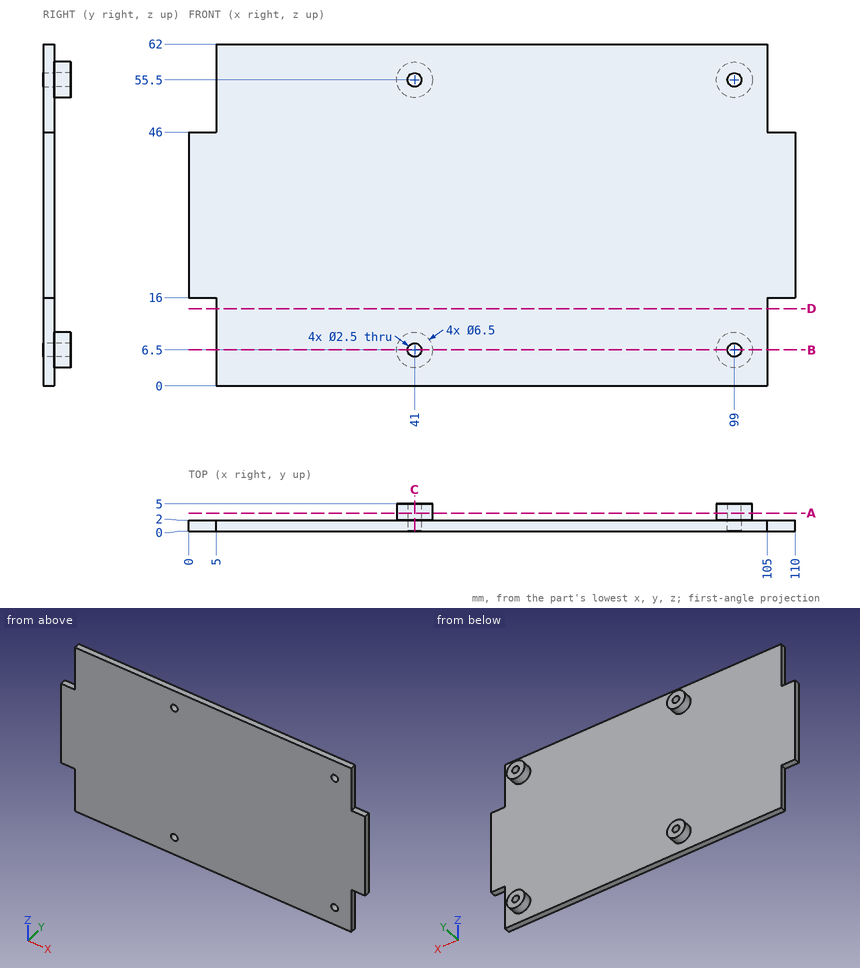
Geometry check sheet. Reference: drawing and pictorial views, mm from the part's lowest x, y, z. Give positions to 0.01 mm unless a question says otherwise; leave off trailing zeros. Order: outer loops, then holes, each group sorted by start corner. A loop starts at its lowest first (then second) coordinate and runs counter-clockwise, first axis right, second up. Notation, with made-up numbers: M -20,48.25 L 10,48.25 A15 cw 10,71.25 Z; hole C -20.75,-20 d2. An arc over 180 degrees is marked long. Answer as CSV lines item,"result". Start each with the question number.
Item 1: Cross-section at A-A on y = 3.3. Enter the section's corners in (x, z).
Item 2: Cross-section at C-C on x = 41. Enter the section's corners in (y, z), plus the area to 3 significant figures.
Item 3: Cross-section at B-B on z = 6.5. Enter the section's corners in (x, y).
Item 4: Gauge pin test, flat ends, axial feed: P1, Ø0.6, axis at y = 1, z = 11, coming from the +X side; P2, Ø3, axis at x = 41, z = 55.5, coming from the +Y side; P3, Ø2, axis at x = 95, z = 35, coming from the +Y side; P4, Ø0.6, axis at x = 3, y = 1.5, coming from the +Z side. Record the tip position at first contact, or that the pin passes through.
Item 5: Cross-section at D-D on z = 14. Enter the section's corners in (x, y).
Item 6: Thickness scan on line 1 (Z direction, x = 41, y = 0.7); line 2 (Z direction, x = 41, y = 3.9); line 3 (X direction, y = 3.3, z = 55.5). Record the ranges inside material, lowest first. Write a range as [from, to].
Established:
1,outline,"C 41,6.5 d6.5; C 41,55.5 d6.5; C 99,6.5 d6.5; C 99,55.5 d6.5; hole C 41,6.5 d2.5; hole C 41,55.5 d2.5; hole C 99,6.5 d2.5; hole C 99,55.5 d2.5"
2,outline,"M 0,0 L 2,0 L 2,3.25 L 5,3.25 L 5,5.25 L 0,5.25 Z; M 0,7.75 L 5,7.75 L 5,9.75 L 2,9.75 L 2,52.25 L 5,52.25 L 5,54.25 L 0,54.25 Z; M 0,56.75 L 5,56.75 L 5,58.75 L 2,58.75 L 2,62 L 0,62 Z"
2,area,"138 mm^2"
3,outline,"M 5,0 L 39.75,0 L 39.75,5 L 37.75,5 L 37.75,2 L 5,2 Z; M 42.25,0 L 97.75,0 L 97.75,5 L 95.75,5 L 95.75,2 L 44.25,2 L 44.25,5 L 42.25,5 Z; M 100.25,0 L 105,0 L 105,2 L 102.25,2 L 102.25,5 L 100.25,5 Z"
4,P1,"stops at x = 105"
4,P2,"stops at y = 5"
4,P3,"stops at y = 2"
4,P4,"stops at z = 46"
5,outline,"M 5,0 L 105,0 L 105,2 L 5,2 Z"
6,line 1,"z = [0, 5.25], [7.75, 54.25], [56.75, 62]"
6,line 2,"z = [3.25, 5.25], [7.75, 9.75], [52.25, 54.25], [56.75, 58.75]"
6,line 3,"x = [37.75, 39.75], [42.25, 44.25], [95.75, 97.75], [100.25, 102.25]"
